Here's how the part is built. I have some questions about the finished solid (model axes, mm). Give positions to 0.01 mm unless a question says otherwise; leave off trailing zeros. Order: outer loops, then holes, each group sorted by start corner. A loop starts at its lowest first (then second) coordinate and runs counter-clockwise, first axis right, second up. Notation, with made-up numbers: (49.25, 30) - (94.25, 30) arc R12 ccw to (94.25, 35) - close; hole circle Ø9 at (51.5, -1). An arc over 180 degrees is marked (long way). One line per question, with ' | ' between items.
from build123d import *

# Parameters (mm, degrees)
F0_R     = 1.5875
F1_DEPTH = 3.048


with BuildPart() as f1:
    # F0 (on Front) → F1 (new body)
    with BuildSketch(Plane.XZ):
        with BuildLine():
            ThreePointArc((2.6743082177, -18.8613513714), (14.3848543883, -12.4891338461), (19.05, 0))
            ThreePointArc((19.05, 0), (0.4763992031, 19.0440422127), (-19.0261725774, 0.9525004235))
            ThreePointArc((-19.0261725774, 0.9525004235), (-13.8030364969, -13.1293062827), (0, -19.05))
            Line((0, -19.05), (2.6743082177, -18.8613513714))
        make_face()
        Circle(F0_R, mode=Mode.SUBTRACT)
        with BuildLine():
            ThreePointArc((-19.0261725774, 0.9525004235), (0.4763992031, 19.0440422127), (19.05, 0))
            Line((19.05, 0), (28.575, 0))
            ThreePointArc((28.575, 0), (33.6330108411, 11.6193102435), (45.5839285714, 15.8344507639))
            Line((45.5839285714, 15.8344507639), (25.1330658708, 17.2989674606))
            ThreePointArc((25.1330658708, 17.2989674606), (20.0143532381, 19.6729228807), (17.7599894, 24.8454200569))
            Line((17.7599894, 24.8454200569), (15.8989821959, 63.3863857925))
            Line((15.8989821959, 63.3863857925), (19.0127565626, 113.109375))
            ThreePointArc((19.0127565626, 113.109375), (0, 95.25), (-19.0127565626, 113.109375))
            Line((-19.0127565626, 113.109375), (-15.8998639519, 63.4004663068))
            Line((-15.8998639519, 63.4004663068), (-19.0261725774, 0.9525004235))
        make_face()
        with Locations((0, 63.5)):
            Circle(F0_R, mode=Mode.SUBTRACT)
        with Locations((-10.4428892955, 92.5013944507)):
            Circle(F0_R, mode=Mode.SUBTRACT)
        with BuildLine():
            Line((28.575, 0), (19.05, 0))
            ThreePointArc((19.05, 0), (14.3848543883, -12.4891338461), (2.6743082177, -18.8613513714))
            Line((2.6743082177, -18.8613513714), (45.5670640422, -15.8356494318))
            ThreePointArc((45.5670640422, -15.8356494318), (33.6268250192, -11.6135484816), (28.575, 0))
        make_face()
        with BuildLine():
            ThreePointArc((45.5839285714, 15.8344507639), (33.6330108411, 11.6193102435), (28.575, 0))
            ThreePointArc((28.575, 0), (33.6268250192, -11.6135484816), (45.5670640422, -15.8356494318))
            ThreePointArc((45.5670640422, -15.8356494318), (56.0635484816, -10.8231749808), (60.325, 0))
            ThreePointArc((60.325, 0), (56.0693102435, 10.8169891589), (45.5839285714, 15.8344507639))
        make_face()
        with BuildLine():
            ThreePointArc((46.0375, 0), (44.45, -1.5875), (42.8625, 0))
            ThreePointArc((42.8625, 0), (44.45, 1.5875), (46.0375, 0))
        make_face(mode=Mode.SUBTRACT)
        with BuildLine():
            ThreePointArc((0, -19.05), (1.3404768506, -19.0027793181), (2.6743082177, -18.8613513714))
            Line((2.6743082177, -18.8613513714), (0, -19.05))
        make_face()
        with BuildLine():
            ThreePointArc((19.05, 114.3), (-0.5956036778, 133.3406868642), (-19.0127565626, 113.109375))
            ThreePointArc((-19.0127565626, 113.109375), (0, 95.25), (19.0127565626, 113.109375))
            ThreePointArc((19.0127565626, 113.109375), (19.0406868642, 113.7043963222), (19.05, 114.3))
        make_face()
        with Locations((0, 114.3)):
            Circle(F0_R, mode=Mode.SUBTRACT)
    extrude(amount=-F1_DEPTH)


solid = f1.part
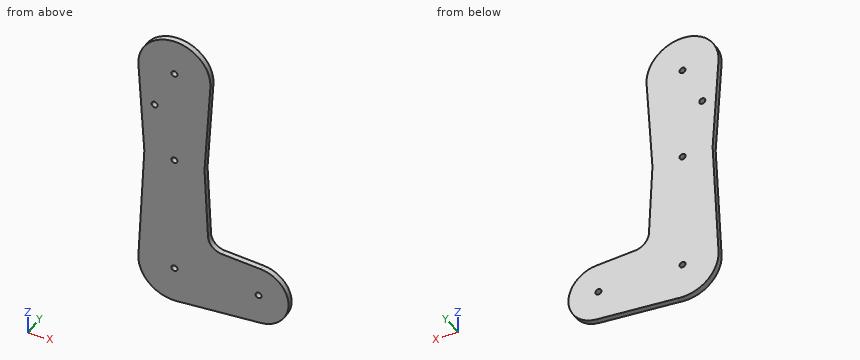
1) Please list where these lines run through material, in increasing order: L1, parallel to Z at x = 44.45, y = 2.4; L2, parallel to Z at x = -14, y = 2.8; L3, parallel to X at y = 2.65, z = 98.5.
Model answer:
L1: z = -15.91 to -1.59, 1.59 to 15.92 | L2: z = -12.92 to 127.22 | L3: x = -18.1 to 18.1
2) I want a section at C-C (x = 22.5). List the corners of the cut face in (y, z) for me.
Model answer:
outline: (0, -17.46) - (3.05, -17.46) - (3.05, 17.95) - (0, 17.95) - close
3) I want a section at A-A (y = 1.5). State how many separate pieces and enclosed holes the cut face has, plus the area to 3 significant figures.
Model answer:
separate pieces: 1 | enclosed holes: 5 | area: 6,430 mm2
4) I want a section at B-B (z = 21.5). List the corners of the cut face in (x, y) for me, plus the area to 3 significant figures.
Model answer:
outline: (-18, 0) - (18.68, 0) - (18.68, 3.05) - (-18, 3.05) - close | area: 112 mm2
